CAD build for the part. Positions are in the model's coordinates, mm. A direction names the side the tool comes from. Coordinates: 2 decimals unless noted, no trailing zeros. Write each loop counter-clockwise with the first axis right and the second up, starting at its lowest first coordinate (ties: lowest second). Pieces come first, ordered by that corner, then holes. Notation, with made-up numbers: (-5, 0) -> (39, 0) arc R11 cw to (39, 8) -> close; hole circle Ø3 at (53.5, -8.75). An arc over 180 degrees is marked (long way). Answer as CSV lines item,"result".
```python
from build123d import *

# Parameters (mm, degrees)
BOSS_EXTRUDE1_DEPTH         = 14
TAP_DRILL_FOR_M4X0_7_TAP2_D = 3.3
F_12_0_12_DIAMETER_HOLE1_D  = 8
TAP_DRILL_FOR_M5X0_8_TAP1_D = 5.5


with BuildPart() as part:
    # Sketch2 → Boss-Extrude1 (new body)
    with BuildSketch(Plane.XY):
        Polygon((-1, 0), (-1, 17.5), (-9, 17.5), (-9, -14), (-21, -14), (-21, -20), (0, -20), (0, 0), align=None)
    boss_extrude1 = extrude(amount=BOSS_EXTRUDE1_DEPTH)

    # Mirror1: Boss-Extrude1 across plane
    add(boss_extrude1.mirror(Plane(origin=(0, -20, 14), x_dir=(0, 0, 1), z_dir=(-1, 0, 0))))

    # Tap Drill for M4x0.7 Tap2 (through all)
    with Locations(Plane.ZY.offset(9)):
        with Locations((7, 10)):
            Hole(TAP_DRILL_FOR_M4X0_7_TAP2_D / 2)

    # Ø12.0 (12) Diameter Hole1 (through all)
    with Locations(Plane(origin=(0, 0, 0), x_dir=(1, 0, 0), z_dir=(0, 0, -1))):
        with Locations((0, 0)):
            Hole(F_12_0_12_DIAMETER_HOLE1_D / 2)

    # Tap Drill for M5x0.8 Tap1 (through all)
    with Locations(Plane(origin=(0, -20, 0), x_dir=(-1, 0, 0), z_dir=(0, -1, 0))):
        with Locations((-16, -7), (16, -7)):
            Hole(TAP_DRILL_FOR_M5X0_8_TAP1_D / 2)


solid = part.part
```
Item 1: 3-axis set-ups, long thin cutter, end or side, ignore diameter. For faces 1 (the flat face through (13.6, -14, 5.3)), 2 (the flat face through (0, -20, 7)), 3 (the flat face through (-13.6, -14, 5.3)), 4 (the flat face through (-5, 17.5, 7)), 5 (the flat face through (-1, 12, 7)): which of +Z, -Z, +X, -X, +Y, -Y reach the whole face in a straight line?
Answer below:
face 1,"+Z, -Z, +X, +Y"
face 2,"+Z, -Z, +X, -X, -Y"
face 3,"+Z, -Z, -X, +Y"
face 4,"+Z, -Z, +X, -X, +Y"
face 5,"+Z, -Z, +Y"
Item 2: Saw through at A-A on x = 16. Give the cut face in (y, z), and give its area (3 significant figures).
Answer below:
outline,"(-20, 0) -> (-14, 0) -> (-14, 4.25) -> (-20, 4.25) -> close; (-20, 9.75) -> (-14, 9.75) -> (-14, 14) -> (-20, 14) -> close"
area,"51.0 mm2"
Item 3: Two-plate mould, pull along X, no slides. Class faces 6 (the cylindrical face through (5.06, 9, 8.31)), 7 (the flat face through (1, 12, 7)), 8 (the flat face through (-9, 2, 7)), 9 (the cylindrical face through (13.818, -16.958, 8.673)): pulls with the +X half, pulls with the -X half, needs draft (parallel to the pull), parting line crosses it, or undercut.
Answer below:
face 6,"needs draft"
face 7,"undercut"
face 8,"pulls with the -X half"
face 9,"undercut"
Item 4: Wall check: line 1 (X direction, y = 6.5, z = 12.25); line 2 (Y direction, x = -6, z = 7); line 3 (X direction, y = 0, z = 8.5). Give the ranges that are in metal, low to high. Write a range as from..to.
Answer below:
line 1,"x = -9..-1, 1..9"
line 2,"y = -20..8.35, 11.65..17.5"
line 3,"x = -9..-4, 4..9"
Item 5: Saw through at B-B on y = 10. Give the cut face in (x, z), and give its area (3 significant figures).
Answer below:
outline,"(-9, 0) -> (-1, 0) -> (-1, 5.35) -> (-9, 5.35) -> close; (-9, 8.65) -> (-1, 8.65) -> (-1, 14) -> (-9, 14) -> close; (1, 0) -> (9, 0) -> (9, 5.35) -> (1, 5.35) -> close; (1, 8.65) -> (9, 8.65) -> (9, 14) -> (1, 14) -> close"
area,"171 mm2"
Item 6: Saw through at C-C on z = 7. Give the cut face in (x, y), and give its area (3 significant figures).
Answer below:
outline,"(-21, -20) -> (-18.75, -20) -> (-18.75, -14) -> (-21, -14) -> close; (-13.25, -20) -> (13.25, -20) -> (13.25, -14) -> (9, -14) -> (9, 8.35) -> (1, 8.35) -> (1, 3.87) arc R4 cw (long way) to (-1, 3.87) -> (-1, 8.35) -> (-9, 8.35) -> (-9, -14) -> (-13.25, -14) -> close; (-9, 11.65) -> (-1, 11.65) -> (-1, 17.5) -> (-9, 17.5) -> close; (1, 11.65) -> (9, 11.65) -> (9, 17.5) -> (1, 17.5) -> close; (18.75, -20) -> (21, -20) -> (21, -14) -> (18.75, -14) -> close"
area,"623 mm2"
Item 7: Flat gauge pins, fed straight in: pin 1 (6 mm diameter, centred on x = 13.5, z = 9.5, fed in from +Y); pin 2 (5.5 mm diameter, centred on y = 10, z = 7, fed in from -X); pin 3 (7 mm diameter, centred on y = -1, z = 7.5, fed in from +X). Where does each tip first touch, or does it go through?
Answer below:
pin 1,"stops at y = -14"
pin 2,"stops at x = -9"
pin 3,"stops at x = 9"
Item 8: Saw through at D-D on x = -7. Give the cut face in (y, z), and give its area (3 significant figures).
Answer below:
outline,"(-20, 0) -> (17.5, 0) -> (17.5, 14) -> (-20, 14) -> close; hole circle Ø3.3 at (10, 7)"
area,"516 mm2"
